Geometry check sheet. Reference: the model listing, model coordinates, mm. A direction names the side the tool comes from. Round coordinates to 2 decimals unless told otherwise and drop trailing zeros. Order: outer loops, then holes, each group sorted by start corner. A loop starts at its lowest first (then second) coordinate and runs counter-clockwise, first axis right, second up. Notation, with made-up numbers: (76.5, 21) - (84.5, 21) arc R30 cw to (84.5, 43) - close; hole circle Ø11 at (-18.5, 10). An arc over 180 degrees is marked (long way). Use a Markdown table: item, result. Add a question column.
(1) Section check A-A on x = -60. Record the boundary of the cut face in (y, z) (3 decimals).
(2) Section check B-B on z = 0. Record the boundary of the cut face in (x, y) (3 decimals).
(3) Section check D-D on x = 0. Record the boundary of the cut face in (y, z).
(4) Thickness scan on line 1 along X through (y, z) = (3, 0) (3 decimals); line 2 along Z through (x, y) = (-60, -3.75) (3 decimals); line 3 along X through (y, z) = (3.25, 3) (3 decimals). Record the ranges inside material, lowest first. Write a range as [from, to].
(5) Gauge pin test, flat ends, axial feed: P1, Ø4, axis at x = -0.5, z = 22, coming from the -Y side; P2, Ø4, axis at y = 2.5, z = 17.5, coming from the +X side; P3, Ø4, axis at y = -1.5, z = -2, coming from the -X side (3 decimals); P4, Ø4, axis at x = 15.5, y = -1.5, coming from the -Z side. Record the tip position at first contact, or that the pin passes through.
(6) Section check C-C on y = -2. Record the boundary of the cut face in (x, z) (3 decimals), then the cut area to 3 significant figures.
(7) Mould release check, pull along Z, two halves, no side actions. Record for faces 1 (the face through (66.32, -0.11, -0.83)), 2 (the face through (-69.37, 0.11, -0.35)), 3 (the face through (0, 0, 29)): released by +Z, released by -Z, zero draft, split by the parting line, or undercut.
(8) Access from +Z, -Z, +X, -X, +Y, -Y to the whole of each face (thin tool, end or side, straight path). Record for faces 4 (the face through (0, -4.5, 22)), 5 (the face through (1, 0, -4)), 6 (the face through (-0.8, 6.2, 16.3)).
```python
from build123d import *

# Parameters (mm, degrees)
SKETCH1_R                            = 9.375
SKETCH1_R_2                          = 6.375
BOSS_EXTRUDE1_DEPTH                  = 7.5
BOSS_EXTRUDE1_2_DEPTH                = 7.5
BOSS_EXTRUDE2_REACH                  = 72.406
BOSS_EXTRUDE2_END_RADIUS             = 9.375
SKETCH2_W                            = 8
SKETCH2_H                            = 15
BOSS_EXTRUDE2_DIRECTION_2_REACH      = 72.406
BOSS_EXTRUDE2_DIRECTION_2_END_RADIUS = 9.375
SKETCH4_R                            = 6.25
BOSS_EXTRUDE3_DEPTH                  = 25
CUT_EXTRUDE1_REACH                   = 77.565
CUT_EXTRUDE1_END_RADIUS              = 6.25
SKETCH5_W                            = 8
SKETCH5_H                            = 3
CUT_EXTRUDE1_DIRECTION_2_REACH       = 77.565
CUT_EXTRUDE1_DIRECTION_2_END_RADIUS  = 6.25


with BuildPart() as part:
    # Sketch1 → Boss-Extrude1 (new, symmetric)
    with BuildSketch(Plane(origin=(0, 0, 0), x_dir=(1, 0, 0), z_dir=(0, 1, 0))):
        with Locations(Location((-60, 0, 0), (0, 0, 90))):
            Circle(SKETCH1_R)
        with Locations(Location((-60, 0, 0), (0, 0, 90))):
            Circle(SKETCH1_R_2, mode=Mode.SUBTRACT)
    extrude(amount=BOSS_EXTRUDE1_DEPTH, both=True)



with BuildPart() as body_2:
    # Sketch1 → Boss-Extrude1 2 (new, symmetric)
    with BuildSketch(Plane(origin=(0, 0, 0), x_dir=(1, 0, 0), z_dir=(0, 1, 0))):
        with Locations(Location((60, 0, 0), (0, 0, 270))):
            Circle(SKETCH1_R)
        with Locations(Location((60, 0, 0), (0, 0, 270))):
            Circle(SKETCH1_R_2, mode=Mode.SUBTRACT)
    extrude(amount=BOSS_EXTRUDE1_2_DEPTH, both=True)


with BuildPart() as part_1:
    add(part.part)

    add(body_2.part)  # Boss-Extrude2 merges body 2
    # Boss-Extrude2: up to this cylinder (the profile starts outside it)
    boss_extrude2_end = Plane(origin=(60, 0, 0), z_dir=(0, -1, 0)) * Cylinder(BOSS_EXTRUDE2_END_RADIUS, 164.562, mode=Mode.PRIVATE)
    # Sketch2 → Boss-Extrude2 (add, up to the surface)
    with BuildSketch(Plane(origin=(0, 0, 0), x_dir=(0, 0, -1), z_dir=(1, 0, 0)), mode=Mode.PRIVATE) as boss_extrude2_sk1:
        Rectangle(SKETCH2_W, SKETCH2_H)
    boss_extrude2_tool1 = extrude(boss_extrude2_sk1.sketch, amount=BOSS_EXTRUDE2_REACH, mode=Mode.PRIVATE) - boss_extrude2_end
    add(boss_extrude2_tool1.solids().sort_by_distance((0, 0, 0))[0])

    # Boss-Extrude2 direction 2: up to this cylinder (the profile starts outside it)
    boss_extrude2_direction_2_end = Plane(origin=(-60, 0, 0), z_dir=(0, -1, 0)) * Cylinder(BOSS_EXTRUDE2_DIRECTION_2_END_RADIUS, 164.562, mode=Mode.PRIVATE)
    # Sketch2 → Boss-Extrude2 direction 2 (add, up to the surface)
    with BuildSketch(Plane(origin=(0, 0, 0), x_dir=(0, 0, -1), z_dir=(1, 0, 0)), mode=Mode.PRIVATE) as boss_extrude2_direction_2_sk1:
        Rectangle(SKETCH2_W, SKETCH2_H)
    boss_extrude2_direction_2_tool1 = extrude(boss_extrude2_direction_2_sk1.sketch, amount=-BOSS_EXTRUDE2_DIRECTION_2_REACH, mode=Mode.PRIVATE) - boss_extrude2_direction_2_end
    add(boss_extrude2_direction_2_tool1.solids().sort_by_distance((0, 0, 0))[0])

    # Sketch4 → Boss-Extrude3 (add)
    with BuildSketch(Plane.XY.offset(4)):
        Circle(SKETCH4_R)
    extrude(amount=BOSS_EXTRUDE3_DEPTH)

    # Cut-Extrude1: up to this cylinder (the profile starts inside it)
    cut_extrude1_end = Plane(origin=(0, 0, 22), z_dir=(0, 0, -1)) * Cylinder(CUT_EXTRUDE1_END_RADIUS, 168.63, mode=Mode.PRIVATE)
    # Sketch5 → Cut-Extrude1 (cut, up to the surface)
    with BuildSketch(Plane(origin=(0, 0, 0), x_dir=(0, 0, -1), z_dir=(1, 0, 0)), mode=Mode.PRIVATE) as cut_extrude1_sk1:
        with Locations((-22, -6)):
            Rectangle(SKETCH5_W, SKETCH5_H)
    cut_extrude1_tool1 = extrude(cut_extrude1_sk1.sketch, amount=-CUT_EXTRUDE1_REACH, mode=Mode.PRIVATE) & cut_extrude1_end
    add(cut_extrude1_tool1.solids().sort_by_distance((0, -6, 22))[0], mode=Mode.SUBTRACT)

    # Cut-Extrude1 direction 2: up to this cylinder (the profile starts inside it)
    cut_extrude1_direction_2_end = Plane(origin=(0, 0, 22), z_dir=(0, 0, -1)) * Cylinder(CUT_EXTRUDE1_DIRECTION_2_END_RADIUS, 168.63, mode=Mode.PRIVATE)
    # Sketch5 → Cut-Extrude1 direction 2 (cut, up to the surface)
    with BuildSketch(Plane(origin=(0, 0, 0), x_dir=(0, 0, -1), z_dir=(1, 0, 0)), mode=Mode.PRIVATE) as cut_extrude1_direction_2_sk1:
        with Locations((-22, -6)):
            Rectangle(SKETCH5_W, SKETCH5_H)
    cut_extrude1_direction_2_tool1 = extrude(cut_extrude1_direction_2_sk1.sketch, amount=CUT_EXTRUDE1_DIRECTION_2_REACH, mode=Mode.PRIVATE) & cut_extrude1_direction_2_end
    add(cut_extrude1_direction_2_tool1.solids().sort_by_distance((0, -6, 22))[0], mode=Mode.SUBTRACT)


solid = part_1.part
```
Check sheet entries:
| question | item | result |
|---|---|---|
| 1 | outline | (-7.5, -9.375) - (7.5, -9.375) - (7.5, -6.375) - (-7.5, -6.375) - close; (-7.5, 6.375) - (7.5, 6.375) - (7.5, 9.375) - (-7.5, 9.375) - close |
| 2 | outline | (-69.375, -7.5) - (-66.375, -7.5) - (-66.375, 7.5) - (-69.375, 7.5) - close; (-53.625, -7.5) - (53.625, -7.5) - (53.625, 7.5) - (-53.625, 7.5) - close; (66.375, -7.5) - (69.375, -7.5) - (69.375, 7.5) - (66.375, 7.5) - close |
| 3 | outline | (-7.5, -4) - (7.5, -4) - (7.5, 4) - (6.25, 4) - (6.25, 29) - (-6.25, 29) - (-6.25, 26) - (-4.5, 26) - (-4.5, 18) - (-6.25, 18) - (-6.25, 4) - (-7.5, 4) - close |
| 4 | line 1 | x = [-69.375, -66.375], [-53.625, 53.625], [66.375, 69.375] |
| 4 | line 2 | z = [-9.375, -6.375], [6.375, 9.375] |
| 4 | line 3 | x = [-68.882, -65.625], [-54.375, 54.375], [65.625, 68.882] |
| 5 | P1 | stops at y = -4.5 |
| 5 | P2 | stops at x = 6.23 |
| 5 | P3 | stops at x = -69.375 |
| 5 | P4 | stops at z = -4 |
| 6 | outline | (-51.521, -4) - (51.521, -4) arc R9.375 ccw (long way) to (51.521, 4) - (5.921, 4) - (5.921, 29) - (-5.921, 29) - (-5.921, 4) - (-51.521, 4) arc R9.375 ccw (long way) to start; hole circle Ø12.75 at (-60, 0); hole circle Ø12.75 at (60, 0) |
| 6 | area | 1,410 mm2 |
| 7 | face 1 | undercut |
| 7 | face 2 | split by the parting line |
| 7 | face 3 | released by +Z |
| 8 | face 4 | +X, -X, -Y |
| 8 | face 5 | -Z, +Y, -Y |
| 8 | face 6 | +Z |
